Geometry check sheet. Reference: drawing and pictorial views, mm from the part's lowest x, y, z. A direction names the side the tool comes from. Round coordinates to 2 decimals unless told otherwise and drop trailing zeros. Loops run counter-clockwise (first coordinate to the right, second up) from the corner with the lowest first, then second, coordinate; pieces in that order, holes last. Notation, with made-up numbers: (72.5, 87) -> (115.5, 87) arc R25 cw to (115.5, 114) -> close; hole circle Ø5 at (85.25, 17). An arc over 180 degrees is marked (long way). Use one line per item in the form item = value.
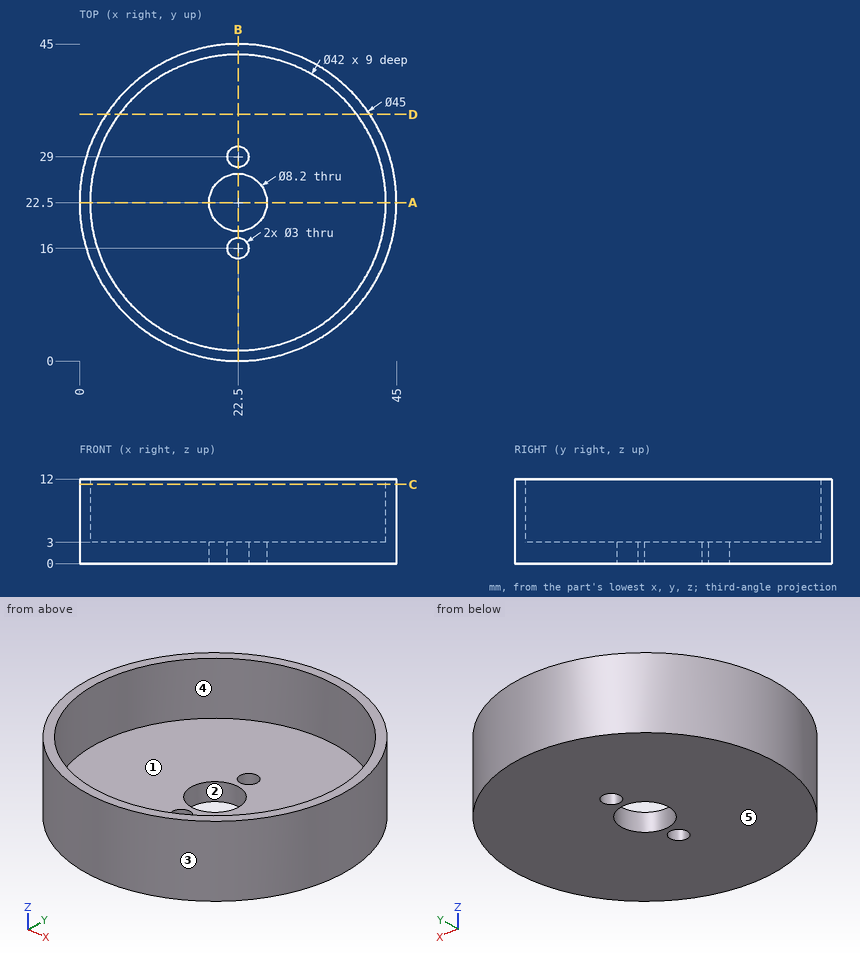
1. Section check B-B (x = 22.5). Record the boundary of the cut face in (y, z).
Return value:
outline = (0, 0) -> (14.5, 0) -> (14.5, 3) -> (1.5, 3) -> (1.5, 12) -> (0, 12) -> close; (17.5, 0) -> (18.4, 0) -> (18.4, 3) -> (17.5, 3) -> close; (26.6, 0) -> (27.5, 0) -> (27.5, 3) -> (26.6, 3) -> close; (30.5, 0) -> (45, 0) -> (45, 12) -> (43.5, 12) -> (43.5, 3) -> (30.5, 3) -> close
2. Gauge pin test, flat ends, axial feed: pin 1 (3 mm diameter, centred on x = 16, y = 27.5, fed in from +Z); pin 2 (4 mm diameter, centred on x = 37, z = 2.5, fed in from +Y); pin 3 (5 mm diameter, centred on y = 28.5, z = 3.5, fed in from +X). Record the tip position at first contact, or that the pin passes through.
Return value:
pin_1 = 3
pin_2 = 41.21
pin_3 = 44.73
3. Tool access check on the marked faces 1 and 2. Record the directions out of +Z, -Z, +X, -X, +Y, -Y that give a thin tool (end or side, any length) a straight path to the whole face; none if there is none.
Return value:
face_1 = +Z
face_2 = +Z, -Z
4. Section check C-C (z = 11.25). Record the boundary of the cut face in (x, y).
Return value:
outline = circle Ø45 at (22.5, 22.5); hole circle Ø42 at (22.5, 22.5)
5. Mould release check, pull along Y, two halves, no side actions. Record for the marked faces 3, 4 and 5: released by +Y, released by -Y, zero draft, split by the parting line, or undercut.
Return value:
face_3 = split by the parting line
face_4 = undercut
face_5 = zero draft
6. Section check A-A (y = 22.5). Record the boundary of the cut face in (x, z).
Return value:
outline = (0, 0) -> (18.4, 0) -> (18.4, 3) -> (1.5, 3) -> (1.5, 12) -> (0, 12) -> close; (26.6, 0) -> (45, 0) -> (45, 12) -> (43.5, 12) -> (43.5, 3) -> (26.6, 3) -> close
7. Section check D-D (y = 35). Record the boundary of the cut face in (x, z), then the cut area to 3 significant figures.
Return value:
outline = (3.79, 0) -> (41.21, 0) -> (41.21, 12) -> (39.37, 12) -> (39.37, 3) -> (5.63, 3) -> (5.63, 12) -> (3.79, 12) -> close
area = 145 mm2
8. Material ranges on line 1 along Y through (x, z) = (22.5, 1.05); line 2 along Y through (x, z) = (22.5, 8); line 3 along Z through (x, y) = (41, 32), recorded low to high.
Return value:
line_1 = 0 to 14.5, 17.5 to 18.4, 26.6 to 27.5, 30.5 to 45
line_2 = 0 to 1.5, 43.5 to 45
line_3 = 0 to 3
